Geometry check sheet. Reference: the model listing, model coordinates, mm. A direction names the side the tool comes from. Round coordinates to 2 decimals unless told otherwise and drop trailing zeros. Order: outer loops, then holes, each group sorted by start corner. A loop starts at its lowest first (then second) coordinate and runs counter-clockwise, first axis right, second up. Notation, with made-up numbers: (-15.5, -19.75) - (16.5, -19.75) arc R34 ccw to (16.5, 16.25) - close; hole circle Ø6 at (54, -20.75). An arc over 180 degrees is marked (long way). Use a Markdown table: item, result. Add a question column.
(1) Thickness scan on line 1 along Z through (x, y) = (13.5, 2.55); line 2 along Z through (x, y) = (80, 1.6); line 3 along Z through (x, y) = (75.5, 2.6). Record the ranges inside material, lowest first. Write a range as [from, to].
(2) Gauge pin test, flat ends, axial feed: P1, Ø2.5, axis at x = 48, z = 0, coming from the +Y side; P2, Ø0.9, axis at x = 14, y = 1.5, coming from the +Z side; P3, Ø0.9, axis at x = 68, y = 1, coming from the -Z side; P4, Ø1, axis at y = 1, z = -2, coming from the -X side. Record the tip position at first contact, or that the pin passes through.
(3) Access from +Z, -Z, +X, -X, +Y, -Y to the whole of each face (thin tool, end or side, straight path). Record for faces 5 (the face through (43, 1, -6)), 6 (the face through (38, 3, 0)), 7 (the face through (70, 1, 0)).
(4) Section check C-C on y = 1.1. Record the boundary of the cut face in (x, z).
(5) Section check B-B on z = 0. Record the boundary of the cut face in (x, y), then the cut area to 3 significant figures.
(6) Mould release check, pull along Z, two halves, no side actions. Record for faces 1 (the face through (42, 1, 6)), 2 (the face through (-7.896, 1.479, -0.243)), 3 (the face through (49.5, 1.48, -0.07)), 4 (the face through (78.8, 1.5, 0.5)): released by +Z, released by -Z, zero draft, split by the parting line, or undercut.
(7) Section check A-A on x = 48. Record the boundary of the cut face in (y, z).
(8) Section check D-D on x = 0. Record the boundary of the cut face in (y, z), then the cut area to 3 significant figures.
```python
from build123d import *

# Parameters (mm, degrees)
RESSALTO_EXTRUS_O1_DEPTH     = 3
ESBO_O2_W                    = 5
ESBO_O2_H                    = 3
ESBO_O2_W_2                  = 7.5
CORTE_EXTRUS_O1_DEPTH        = 87.414177078
FURO_DE_DI_METRO_3_0_3_1_D   = 3
FURO_DE_DI_METRO_2_6_2_6_1_D = 2.6
FILETE1_R                    = 2


with BuildPart() as part:
    # Esboço1 → Ressalto-extrusão1 (new body)
    with BuildSketch(Plane(origin=(0, 0, 0), x_dir=(1, 0, 0), z_dir=(0, 1, 0))):
        with BuildLine():
            Line((80, 6), (5.139066063, 6))
            ThreePointArc((5.139066063, 6), (-7.9, 0), (5.139066063, -6))
            Line((5.139066063, -6), (80, -6))
            ThreePointArc((80, -6), (86, 0), (80, 6))
        make_face()
    extrude(amount=RESSALTO_EXTRUS_O1_DEPTH)

    # Esboço2 → Corte-extrusão1 (cut, through all)
    with BuildSketch(Plane(origin=(0, 0, 0), x_dir=(1, 0, 0), z_dir=(0, 1, 0))):
        with Locations((67.5, 0)):
            Rectangle(ESBO_O2_W, ESBO_O2_H)
        with Locations((13.75, 0)):
            Rectangle(ESBO_O2_W_2, ESBO_O2_H)
    extrude(amount=CORTE_EXTRUS_O1_DEPTH, mode=Mode.SUBTRACT)

    # Furo de diâmetro Ø3.0 (3)1 (through all)
    with Locations(Plane(origin=(0, 3, 0), x_dir=(1, 0, 0), z_dir=(0, 1, 0))):
        with Locations((0, 0), (48, 0)):
            Hole(FURO_DE_DI_METRO_3_0_3_1_D / 2)

    # Furo de diâmetro Ø2.6 (2.6)1 (through all)
    with Locations(Plane(origin=(0, 3, 0), x_dir=(1, 0, 0), z_dir=(0, 1, 0))):
        with Locations((80, 0)):
            Hole(FURO_DE_DI_METRO_2_6_2_6_1_D / 2)

    # Filete1
    filete1_edges = [part.edges().sort_by_distance(p)[0] for p in [
        (5.139066063, 1.5, 6),
        (5.139066063, 1.5, -6),
    ]]
    fillet(filete1_edges, radius=FILETE1_R)


solid = part.part
```
Check sheet entries:
| question | item | result |
|---|---|---|
| 1 | line 1 | z = [-6, -1.5], [1.5, 6] |
| 1 | line 2 | z = [-6, -1.3], [1.3, 6] |
| 1 | line 3 | z = [-6, 6] |
| 2 | P1 | passes through |
| 2 | P2 | stops at z = 6 |
| 2 | P3 | stops at z = -6 |
| 2 | P4 | stops at x = -7.76 |
| 3 | face 5 | -Z, +X, +Y, -Y |
| 3 | face 6 | +Z, -Z, +X, -X, +Y |
| 3 | face 7 | +Y, -Y |
| 4 | outline | (4.65, -6.38) arc R2 cw to (5.83, -6) - (80, -6) arc R6 ccw to (80, 6) - (5.83, 6) arc R2 cw to (4.65, 6.38) arc R7.9 ccw (long way) to start; hole circle Ø3 at (0, 0); hole (10, -1.5) - (17.5, -1.5) - (17.5, 1.5) - (10, 1.5) - close; hole circle Ø3 at (48, 0); hole (65, -1.5) - (70, -1.5) - (70, 1.5) - (65, 1.5) - close; hole circle Ø2.6 at (80, 0) |
| 5 | outline | (-7.9, 0) - (-1.5, 0) - (-1.5, 3) - (-7.9, 3) - close; (1.5, 0) - (10, 0) - (10, 3) - (1.5, 3) - close; (17.5, 0) - (46.5, 0) - (46.5, 3) - (17.5, 3) - close; (49.5, 0) - (65, 0) - (65, 3) - (49.5, 3) - close; (70, 0) - (78.7, 0) - (78.7, 3) - (70, 3) - close; (81.3, 0) - (86, 0) - (86, 3) - (81.3, 3) - close |
| 5 | area | 218 mm2 |
| 6 | face 1 | released by +Z |
| 6 | face 2 | split by the parting line |
| 6 | face 3 | undercut |
| 6 | face 4 | undercut |
| 7 | outline | (0, -6) - (3, -6) - (3, -1.5) - (0, -1.5) - close; (0, 1.5) - (3, 1.5) - (3, 6) - (0, 6) - close |
| 8 | outline | (0, -7.9) - (3, -7.9) - (3, -1.5) - (0, -1.5) - close; (0, 1.5) - (3, 1.5) - (3, 7.9) - (0, 7.9) - close |
| 8 | area | 38.4 mm2 |
